Check sheet for the modelled part. Datum: model origin and axes. Units: mm. Round coordinates to 2 decimals unless told otherwise and drop trailing zeros. Loops run counter-clockwise (first coordinate to the right, second up) from the corner with the lowest first, then second, coordinate; pieces in that order, holes last. Notation, with made-up numbers: (-34.75, -25.5) -> (-20.75, -25.5) arc R28 cw to (-20.75, 7.5) -> close; hole circle Ø7 at (-13.75, 7). An arc over 180 degrees is marked (long way). One line per question, with ' | ' between items.
```python
from build123d import *

# Parameters (mm, degrees)
PAD004_DEPTH    = 1.6
SKETCH010_W     = 13.95
SKETCH010_H     = 13.95
POCKET004_DEPTH = 1.6
SKETCH013_W     = 17
SKETCH013_H     = 14
POCKET005_DEPTH = 1.6


with BuildPart() as part:
    # Sketch008 → Pad004 (new body)
    with BuildSketch(Plane.XY.offset(9.9)):
        Polygon((25.3, 104.99), (143.71, 104.99), (143.71, 102.74), (146.96, 102.74), (146.96, 4.55), (143.71, 4.55), (143.71, 2.3), (5.55, 2.3), (5.55, 4.55), (2.3, 4.55), (2.3, 82.49), (25.3, 82.49), align=None)
    extrude(amount=PAD004_DEPTH)

    # Sketch010 (on Face13 of Pad004) → Pocket004 (cut)
    with BuildSketch(Plane(origin=(0, 0, 9.9), x_dir=(1, 0, 0), z_dir=(0, 0, -1))):
        with Locations((131.78, -16.525)):
            Rectangle(SKETCH010_W, SKETCH010_H)
        with Locations((55.58, -16.525)):
            Rectangle(SKETCH010_W, SKETCH010_H)
        with Locations((36.53, -16.525)):
            Rectangle(SKETCH010_W, SKETCH010_H)
        with Locations((17.48, -16.525)):
            Rectangle(SKETCH010_W, SKETCH010_H)
        with Locations((131.78, -35.575)):
            Rectangle(SKETCH010_W, SKETCH010_H)
        with Locations((112.73, -35.575)):
            Rectangle(SKETCH010_W, SKETCH010_H)
        with Locations((93.68, -35.575)):
            Rectangle(SKETCH010_W, SKETCH010_H)
        with Locations((74.63, -35.575)):
            Rectangle(SKETCH010_W, SKETCH010_H)
        with Locations((55.58, -35.575)):
            Rectangle(SKETCH010_W, SKETCH010_H)
        with Locations((36.53, -35.575)):
            Rectangle(SKETCH010_W, SKETCH010_H)
        with Locations((17.48, -35.575)):
            Rectangle(SKETCH010_W, SKETCH010_H)
        with Locations((131.78, -54.625)):
            Rectangle(SKETCH010_W, SKETCH010_H)
        with Locations((112.73, -54.625)):
            Rectangle(SKETCH010_W, SKETCH010_H)
        with Locations((93.68, -54.625)):
            Rectangle(SKETCH010_W, SKETCH010_H)
        with Locations((74.63, -54.625)):
            Rectangle(SKETCH010_W, SKETCH010_H)
        with Locations((55.58, -54.625)):
            Rectangle(SKETCH010_W, SKETCH010_H)
        with Locations((36.53, -54.625)):
            Rectangle(SKETCH010_W, SKETCH010_H)
        with Locations((17.48, -54.625)):
            Rectangle(SKETCH010_W, SKETCH010_H)
        with Locations((131.78, -73.675)):
            Rectangle(SKETCH010_W, SKETCH010_H)
        with Locations((112.73, -73.675)):
            Rectangle(SKETCH010_W, SKETCH010_H)
        with Locations((93.68, -73.675)):
            Rectangle(SKETCH010_W, SKETCH010_H)
        with Locations((74.63, -73.675)):
            Rectangle(SKETCH010_W, SKETCH010_H)
        with Locations((55.58, -73.675)):
            Rectangle(SKETCH010_W, SKETCH010_H)
        with Locations((36.53, -73.675)):
            Rectangle(SKETCH010_W, SKETCH010_H)
        with Locations((17.48, -73.675)):
            Rectangle(SKETCH010_W, SKETCH010_H)
        with Locations((131.78, -92.725)):
            Rectangle(SKETCH010_W, SKETCH010_H)
        with Locations((112.73, -92.725)):
            Rectangle(SKETCH010_W, SKETCH010_H)
        with Locations((93.68, -92.725)):
            Rectangle(SKETCH010_W, SKETCH010_H)
        with Locations((74.63, -92.725)):
            Rectangle(SKETCH010_W, SKETCH010_H)
        with Locations((55.58, -92.725)):
            Rectangle(SKETCH010_W, SKETCH010_H)
        with Locations((36.53, -92.725)):
            Rectangle(SKETCH010_W, SKETCH010_H)
        with Locations((112.73, -16.525)):
            Rectangle(SKETCH010_W, SKETCH010_H)
    extrude(amount=-POCKET004_DEPTH, mode=Mode.SUBTRACT)

    # Sketch013 (on Face5 of Pocket004) → Pocket005 (cut)
    with BuildSketch(Plane.XY.offset(11.5)):
        with Locations((84.055, 16.6)):
            Rectangle(SKETCH013_W, SKETCH013_H)
    extrude(amount=-POCKET005_DEPTH, mode=Mode.SUBTRACT)


solid = part.part
```
(1) Sectioned sample at A-A, the plane y = 97.5. Record the cut outline in (x, z) (3 decimals).
Answer:
outline: (25.3, 9.9) -> (29.555, 9.9) -> (29.555, 11.5) -> (25.3, 11.5) -> close; (43.505, 9.9) -> (48.605, 9.9) -> (48.605, 11.5) -> (43.505, 11.5) -> close; (62.555, 9.9) -> (67.655, 9.9) -> (67.655, 11.5) -> (62.555, 11.5) -> close; (81.605, 9.9) -> (86.705, 9.9) -> (86.705, 11.5) -> (81.605, 11.5) -> close; (100.655, 9.9) -> (105.755, 9.9) -> (105.755, 11.5) -> (100.655, 11.5) -> close; (119.705, 9.9) -> (124.805, 9.9) -> (124.805, 11.5) -> (119.705, 11.5) -> close; (138.755, 9.9) -> (146.96, 9.9) -> (146.96, 11.5) -> (138.755, 11.5) -> close
(2) Scan lines: probe 1 along Y at (x, z) = (116, 11.3); probe 2 along Y at (x, z) = (95.5, 10.3); probe 3 along Y at (x, z) = (15.5, 10.35). Record each from-to range of solid material in increasing order.
Answer:
probe 1: y = 2.3 to 9.55, 23.5 to 28.6, 42.55 to 47.65, 61.6 to 66.7, 80.65 to 85.75, 99.7 to 104.99 | probe 2: y = 2.3 to 28.6, 42.55 to 47.65, 61.6 to 66.7, 80.65 to 85.75, 99.7 to 104.99 | probe 3: y = 2.3 to 9.55, 23.5 to 28.6, 42.55 to 47.65, 61.6 to 66.7, 80.65 to 82.49
(3) Sectioned sample at C-C, the plane x = 130.5. Record the cut outline in (y, z), and give its area (3 significant figures).
Answer:
outline: (2.3, 9.9) -> (9.55, 9.9) -> (9.55, 11.5) -> (2.3, 11.5) -> close; (23.5, 9.9) -> (28.6, 9.9) -> (28.6, 11.5) -> (23.5, 11.5) -> close; (42.55, 9.9) -> (47.65, 9.9) -> (47.65, 11.5) -> (42.55, 11.5) -> close; (61.6, 9.9) -> (66.7, 9.9) -> (66.7, 11.5) -> (61.6, 11.5) -> close; (80.65, 9.9) -> (85.75, 9.9) -> (85.75, 11.5) -> (80.65, 11.5) -> close; (99.7, 9.9) -> (104.99, 9.9) -> (104.99, 11.5) -> (99.7, 11.5) -> close | area: 52.7 mm2
(4) Sectioned sample at B-B, the plane x = 94.5. Record the cut outline in (y, z), and give its area (3 significant figures).
Answer:
outline: (2.3, 9.9) -> (28.6, 9.9) -> (28.6, 11.5) -> (2.3, 11.5) -> close; (42.55, 9.9) -> (47.65, 9.9) -> (47.65, 11.5) -> (42.55, 11.5) -> close; (61.6, 9.9) -> (66.7, 9.9) -> (66.7, 11.5) -> (61.6, 11.5) -> close; (80.65, 9.9) -> (85.75, 9.9) -> (85.75, 11.5) -> (80.65, 11.5) -> close; (99.7, 9.9) -> (104.99, 9.9) -> (104.99, 11.5) -> (99.7, 11.5) -> close | area: 75.0 mm2
(5) Sectioned sample at D-D, the plane y = 70. Count the separate pieces of the cut face and the enclosed holes in it, and give its area (3 significant figures).
Answer:
separate pieces: 8 | enclosed holes: 0 | area: 75.2 mm2
